CAD build for the part. Positions are in the model's coordinates, mm. Face numbers are marked on the shaded views. Coordinates: 2 decimals unless noted, no trailing zeros. Loops run counter-clockwise (first coordinate to the right, second up) from the corner with the lowest first, then second, coordinate; pieces in that order, holes last. Notation, with made-up numbers: (61.5, 77.25) -> (117.5, 77.25) arc R16 cw to (117.5, 95.25) -> close; hole circle Ø2 at (-34.75, 77). An arc over 180 degrees is marked (long way). Answer as CSV lines item,"result". Start each with the question number.
```python
from build123d import *

# Parameters (mm, degrees)
ESQUISSE1_W             = 50
ESQUISSE1_H             = 40
BOSS_EXTRU_1_DEPTH      = 5
ESQUISSE2_R             = 1.5
ESQUISSE2_R_2           = 3.5
ENL_V_MAT_EXTRU_1_DEPTH = 10


with BuildPart() as part:
    # Esquisse1 → Boss.-Extru.1 (new body)
    with BuildSketch(Plane.XY):
        Rectangle(ESQUISSE1_W, ESQUISSE1_H)
    extrude(amount=BOSS_EXTRU_1_DEPTH)

    # Esquisse2 → Enlèv. mat.-Extru.1 (cut)
    with BuildSketch(Plane(origin=(0, 0, 0), x_dir=(-1, 0, 0), z_dir=(0, 0, -1))):
        with Locations((-8.5, 0)):
            Circle(ESQUISSE2_R)
        with Locations((8.5, 0)):
            Circle(ESQUISSE2_R)
        Circle(ESQUISSE2_R_2)
    extrude(amount=-ENL_V_MAT_EXTRU_1_DEPTH, mode=Mode.SUBTRACT)


solid = part.part
```
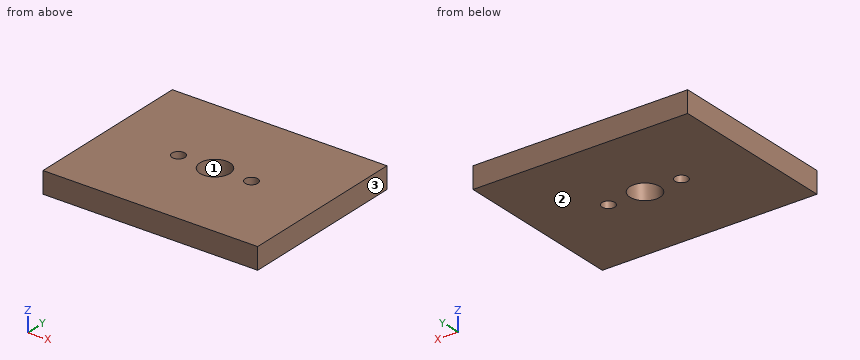
Q1. Saw through at A-A (x = 8.5). List the corners of the cut face in (y, z), and give its area (3 significant figures).
Q2. Saw through at B-B (y = 0). List the corners of the cut face in (x, z).
Q3. Two-plate mould, pull along X, no slides. Class the marked faces 1, 2 and 3: pulls with the +X half, pulls with the -X half, needs draft (parallel to the pull), parting line crosses it, or undercut.
Q4. Saw through at C-C (z = 0.65). List the corners of the cut face in (x, y).
Q5. Saw through at D-D (x = 0). List the corners of the cut face in (y, z).
Q6. Probe probe 1 along Y at (x, z) = (0, 2.45); probe 2 along X at (y, z) = (-0.5, 2.3); probe 3 along Y at (x, z) = (-8.5, 1.85). List the from-to ranges inside material, lowest first. Write a range as from..to.
Ans:
1,outline,"(-20, 0) -> (-1.5, 0) -> (-1.5, 5) -> (-20, 5) -> close; (1.5, 0) -> (20, 0) -> (20, 5) -> (1.5, 5) -> close"
1,area,"185 mm²"
2,outline,"(-25, 0) -> (-10, 0) -> (-10, 5) -> (-25, 5) -> close; (-7, 0) -> (-3.5, 0) -> (-3.5, 5) -> (-7, 5) -> close; (3.5, 0) -> (7, 0) -> (7, 5) -> (3.5, 5) -> close; (10, 0) -> (25, 0) -> (25, 5) -> (10, 5) -> close"
3,face 1,"undercut"
3,face 2,"needs draft"
3,face 3,"pulls with the +X half"
4,outline,"(-25, -20) -> (25, -20) -> (25, 20) -> (-25, 20) -> close; hole circle Ø3 at (-8.5, 0); hole circle Ø7 at (0, 0); hole circle Ø3 at (8.5, 0)"
5,outline,"(-20, 0) -> (-3.5, 0) -> (-3.5, 5) -> (-20, 5) -> close; (3.5, 0) -> (20, 0) -> (20, 5) -> (3.5, 5) -> close"
6,probe 1,"y = -20..-3.5, 3.5..20"
6,probe 2,"x = -25..-9.91, -7.09..-3.46, 3.46..7.09, 9.91..25"
6,probe 3,"y = -20..-1.5, 1.5..20"
